Build history of the part. All positions in model axes, mm. Round coordinates to 2 decimals unless told otherwise and drop trailing zeros. Order: outer loops, then holes, each group sorted by start corner. A loop starts at its lowest first (then second) coordinate and runs counter-clockwise, first axis right, second up. Notation, with made-up numbers: (36.25, 68.5) -> (42.25, 68.5) arc R9 ccw to (42.25, 78.5) -> close; hole circle Ø7 at (-12, 1.5). An arc over 180 degrees is marked (long way). Write item = value, one per line.
from build123d import *

# Parameters (mm, degrees)
SKETCH1_W           = 76.2
SKETCH1_H           = 50.8
SKETCH1_R           = 1.778
BOSS_EXTRUDE1_DEPTH = 1.778
SKETCH2_R           = 0.889
CUT_EXTRUDE1_DEPTH  = 2.778


with BuildPart() as part:
    # Sketch1 → Boss-Extrude1 (new body)
    with BuildSketch(Plane.XY):
        Rectangle(SKETCH1_W, SKETCH1_H)
        with Locations((-34.29, 21.59)):
            Circle(SKETCH1_R, mode=Mode.SUBTRACT)
        with Locations((-34.29, -21.59)):
            Circle(SKETCH1_R, mode=Mode.SUBTRACT)
        with Locations((34.29, 21.59)):
            Circle(SKETCH1_R, mode=Mode.SUBTRACT)
        with Locations((34.29, -21.59)):
            Circle(SKETCH1_R, mode=Mode.SUBTRACT)
    extrude(amount=BOSS_EXTRUDE1_DEPTH)

    # Sketch2 → Cut-Extrude1 (cut, through all)
    with BuildSketch(Plane(origin=(0, 0, 0), x_dir=(-1, 0, 0), z_dir=(0, 0, -1))):
        with Locations((27.420334743, 15.353983533)):
            Circle(SKETCH2_R)
        with Locations((32.500334743, 15.353983533)):
            Circle(SKETCH2_R)
        with Locations((27.420334743, 10.273983533)):
            Circle(SKETCH2_R)
        with Locations((32.500334743, 10.273983533)):
            Circle(SKETCH2_R)
        with Locations((17.260334743, 15.353983533)):
            Circle(SKETCH2_R)
        with Locations((22.340334743, 15.353983533)):
            Circle(SKETCH2_R)
        with Locations((17.260334743, 10.273983533)):
            Circle(SKETCH2_R)
        with Locations((22.340334743, 10.273983533)):
            Circle(SKETCH2_R)
        with Locations((17.260334743, 5.193983533)):
            Circle(SKETCH2_R)
        with Locations((22.340334743, 5.193983533)):
            Circle(SKETCH2_R)
        with Locations((17.260334743, 0.113983533)):
            Circle(SKETCH2_R)
        with Locations((22.340334743, 0.113983533)):
            Circle(SKETCH2_R)
        with Locations((7.100334743, 15.353983533)):
            Circle(SKETCH2_R)
        with Locations((12.180334743, 15.353983533)):
            Circle(SKETCH2_R)
        with Locations((7.100334743, 10.273983533)):
            Circle(SKETCH2_R)
        with Locations((12.180334743, 10.273983533)):
            Circle(SKETCH2_R)
        with Locations((7.100334743, 5.193983533)):
            Circle(SKETCH2_R)
        with Locations((12.180334743, 5.193983533)):
            Circle(SKETCH2_R)
        with Locations((7.100334743, 0.113983533)):
            Circle(SKETCH2_R)
        with Locations((12.180334743, 0.113983533)):
            Circle(SKETCH2_R)
        with Locations((-3.059665257, 15.353983533)):
            Circle(SKETCH2_R)
        with Locations((2.020334743, 15.353983533)):
            Circle(SKETCH2_R)
        with Locations((27.420334743, 5.193983533)):
            Circle(SKETCH2_R)
        with Locations((32.500334743, 5.193983533)):
            Circle(SKETCH2_R)
        with Locations((27.420334743, 0.113983533)):
            Circle(SKETCH2_R)
        with Locations((32.500334743, 0.113983533)):
            Circle(SKETCH2_R)
        with Locations((-3.059665257, 10.273983533)):
            Circle(SKETCH2_R)
        with Locations((2.020334743, 10.273983533)):
            Circle(SKETCH2_R)
        with Locations((-3.059665257, 5.193983533)):
            Circle(SKETCH2_R)
        with Locations((2.020334743, 5.193983533)):
            Circle(SKETCH2_R)
        with Locations((-3.059665257, 0.113983533)):
            Circle(SKETCH2_R)
        with Locations((2.020334743, 0.113983533)):
            Circle(SKETCH2_R)
        with Locations((-13.219665257, 15.353983533)):
            Circle(SKETCH2_R)
        with Locations((-8.139665257, 15.353983533)):
            Circle(SKETCH2_R)
        with Locations((-13.219665257, 10.273983533)):
            Circle(SKETCH2_R)
        with Locations((-8.139665257, 10.273983533)):
            Circle(SKETCH2_R)
        with Locations((-13.219665257, 5.193983533)):
            Circle(SKETCH2_R)
        with Locations((-8.139665257, 5.193983533)):
            Circle(SKETCH2_R)
        with Locations((-13.219665257, 0.113983533)):
            Circle(SKETCH2_R)
        with Locations((-8.139665257, 0.113983533)):
            Circle(SKETCH2_R)
        with Locations((-23.379665257, 15.353983533)):
            Circle(SKETCH2_R)
        with Locations((-18.299665257, 15.353983533)):
            Circle(SKETCH2_R)
        with Locations((-23.379665257, 10.273983533)):
            Circle(SKETCH2_R)
        with Locations((-18.299665257, 10.273983533)):
            Circle(SKETCH2_R)
        with Locations((-23.379665257, 5.193983533)):
            Circle(SKETCH2_R)
        with Locations((-18.299665257, 5.193983533)):
            Circle(SKETCH2_R)
        with Locations((-23.379665257, 0.113983533)):
            Circle(SKETCH2_R)
        with Locations((-18.299665257, 0.113983533)):
            Circle(SKETCH2_R)
        with Locations((-33.539665257, 15.353983533)):
            Circle(SKETCH2_R)
        with Locations((-28.459665257, 15.353983533)):
            Circle(SKETCH2_R)
        with Locations((-33.539665257, 10.273983533)):
            Circle(SKETCH2_R)
        with Locations((-28.459665257, 10.273983533)):
            Circle(SKETCH2_R)
        with Locations((-33.539665257, 5.193983533)):
            Circle(SKETCH2_R)
        with Locations((-28.459665257, 5.193983533)):
            Circle(SKETCH2_R)
        with Locations((-33.539665257, 0.113983533)):
            Circle(SKETCH2_R)
        with Locations((-28.459665257, 0.113983533)):
            Circle(SKETCH2_R)
        with Locations((-28.459665257, -5.193983533)):
            Circle(SKETCH2_R)
        with Locations((-33.539665257, -5.193983533)):
            Circle(SKETCH2_R)
        with Locations((-28.459665257, -10.273983533)):
            Circle(SKETCH2_R)
        with Locations((-33.539665257, -10.273983533)):
            Circle(SKETCH2_R)
        with Locations((-28.459665257, -15.353983533)):
            Circle(SKETCH2_R)
        with Locations((-33.539665257, -15.353983533)):
            Circle(SKETCH2_R)
        with Locations((-18.299665257, -5.193983533)):
            Circle(SKETCH2_R)
        with Locations((-23.379665257, -5.193983533)):
            Circle(SKETCH2_R)
        with Locations((-18.299665257, -10.273983533)):
            Circle(SKETCH2_R)
        with Locations((-23.379665257, -10.273983533)):
            Circle(SKETCH2_R)
        with Locations((-18.299665257, -15.353983533)):
            Circle(SKETCH2_R)
        with Locations((-23.379665257, -15.353983533)):
            Circle(SKETCH2_R)
        with Locations((-8.139665257, -5.193983533)):
            Circle(SKETCH2_R)
        with Locations((-13.219665257, -5.193983533)):
            Circle(SKETCH2_R)
        with Locations((-8.139665257, -10.273983533)):
            Circle(SKETCH2_R)
        with Locations((-13.219665257, -10.273983533)):
            Circle(SKETCH2_R)
        with Locations((-8.139665257, -15.353983533)):
            Circle(SKETCH2_R)
        with Locations((-13.219665257, -15.353983533)):
            Circle(SKETCH2_R)
        with Locations((2.020334743, -5.193983533)):
            Circle(SKETCH2_R)
        with Locations((-3.059665257, -5.193983533)):
            Circle(SKETCH2_R)
        with Locations((2.020334743, -10.273983533)):
            Circle(SKETCH2_R)
        with Locations((-3.059665257, -10.273983533)):
            Circle(SKETCH2_R)
        with Locations((32.500334743, -5.193983533)):
            Circle(SKETCH2_R)
        with Locations((27.420334743, -5.193983533)):
            Circle(SKETCH2_R)
        with Locations((2.020334743, -15.353983533)):
            Circle(SKETCH2_R)
        with Locations((-3.059665257, -15.353983533)):
            Circle(SKETCH2_R)
        with Locations((12.180334743, -5.193983533)):
            Circle(SKETCH2_R)
        with Locations((7.100334743, -5.193983533)):
            Circle(SKETCH2_R)
        with Locations((12.180334743, -10.273983533)):
            Circle(SKETCH2_R)
        with Locations((7.100334743, -10.273983533)):
            Circle(SKETCH2_R)
        with Locations((12.180334743, -15.353983533)):
            Circle(SKETCH2_R)
        with Locations((7.100334743, -15.353983533)):
            Circle(SKETCH2_R)
        with Locations((22.340334743, -5.193983533)):
            Circle(SKETCH2_R)
        with Locations((17.260334743, -5.193983533)):
            Circle(SKETCH2_R)
        with Locations((22.340334743, -10.273983533)):
            Circle(SKETCH2_R)
        with Locations((17.260334743, -10.273983533)):
            Circle(SKETCH2_R)
        with Locations((22.340334743, -15.353983533)):
            Circle(SKETCH2_R)
        with Locations((17.260334743, -15.353983533)):
            Circle(SKETCH2_R)
        with Locations((32.500334743, -10.273983533)):
            Circle(SKETCH2_R)
        with Locations((27.420334743, -10.273983533)):
            Circle(SKETCH2_R)
        with Locations((32.500334743, -15.353983533)):
            Circle(SKETCH2_R)
        with Locations((27.420334743, -15.353983533)):
            Circle(SKETCH2_R)
    extrude(amount=-CUT_EXTRUDE1_DEPTH, mode=Mode.SUBTRACT)


solid = part.part
Q1. Cut at C-C, the plane z = 0.7. Give the number of separate pieces and of enclosed holes in the cut face, and give its area (3 significant figures).
Check values:
separate_pieces = 1
enclosed_holes = 102
area = 3,590 mm²
Q2. Flat gauge pin, fed straight in: pin 1 (1.6 mm diameter, centred on x = -22.34, y = 10.27, fed in from +Z). Where does the tip first touch, or does it go through?
Check values:
pin_1 = through
Q3. Cut at B-B, the plane x = -34.29. List the corners of the cut face in (y, z).
Check values:
outline = (-25.4, 0) -> (-23.37, 0) -> (-23.37, 1.78) -> (-25.4, 1.78) -> close; (-19.81, 0) -> (19.81, 0) -> (19.81, 1.78) -> (-19.81, 1.78) -> close; (23.37, 0) -> (25.4, 0) -> (25.4, 1.78) -> (23.37, 1.78) -> close
Q4. Mould opens along X. For faces 1 (the face through (29.348, -5.155, 0.877)), 2 (the face through (-11.47, -10.81, 0.88)) say: released by +X, released by -X, zero draft, split by the parting line, or undercut.
Check values:
face_1 = undercut
face_2 = undercut
Q5. Cut at A-A, the plane y = -21.59. List the corners of the cut face in (x, z), and give its area (3 significant figures).
Check values:
outline = (-38.1, 0) -> (-36.07, 0) -> (-36.07, 1.78) -> (-38.1, 1.78) -> close; (-32.51, 0) -> (32.51, 0) -> (32.51, 1.78) -> (-32.51, 1.78) -> close; (36.07, 0) -> (38.1, 0) -> (38.1, 1.78) -> (36.07, 1.78) -> close
area = 123 mm²
Q6. Probe probe 1 along X at (y, z) = (-22, 1.2). List the from-to ranges inside material, lowest first.
Check values:
probe_1 = -38.1 to -36.02, -32.56 to 32.56, 36.02 to 38.1
